Model file for the job. Use its own axes, mm. Give positions to 0.01 mm unless a question says otherwise; leave off trailing zeros. Loops run counter-clockwise (first coordinate to the right, second up) from the corner with the lowest first, then second, coordinate; pieces in that order, holes last. Notation, with made-up numbers: M 65.5,-20.5 L 94.5,-20.5 A23 ccw 94.5,4.5 Z; hole C -27,52 d8. An arc over 180 degrees is marked long. Use CSV: the item, a comma, the result in double quotes. Start each with the question number.
(1) Slice it at A-A on x = 0. List the corners of the cut face in (y, z), and give its area (3 significant figures).
(2) Slice it at B-B on z = -36. List the corners of the cut face in (x, y).
(3) Slice it at C-C on y = 22. List the corners of the cut face in (x, z).
(4) Wall check: line 1 along X through (y, z) = (64.5, 0); line 2 along Z through (x, y) = (54, 66); line 3 along Z through (x, y) = (-15, 9.5). Give the ranges that are in metal, low to high. Write a range as from..to.
(5) Two-plate mould, pull along X, no slides. Class faces 1 (the face through (-1, 99, -456)), 2 (the face through (-51.721, 50.193, -67.453)), 3 (the face through (-100, 49, -355)): pulls with the +X half, pulls with the -X half, needs draft (parallel to the pull), parting line crosses it, or undercut.
```python
from build123d import *

# Parameters (mm, degrees)
BOSS_EXTRUDE1_DEPTH = 99
SKETCH2_R           = 85
CUT_EXTRUDE1_DEPTH  = 99


with BuildPart() as part:
    # Sketch1 → Boss-Extrude1 (new body)
    with BuildSketch(Plane(origin=(0, 0, 0), x_dir=(1, 0, 0), z_dir=(0, 1, 0))):
        with BuildLine():
            ThreePointArc((-100, 0), (0, -100), (100, 0))
            Line((100, 0), (-100, 0))
        make_face()
        with BuildLine():
            Line((-100, 0), (100, 0))
            ThreePointArc((100, 0), (0, 100), (-100, 0))
        make_face()
        with BuildLine():
            ThreePointArc((-100, 0), (0, 100), (100, 0))
            Line((100, 0), (100, 700))
            ThreePointArc((100, 700), (0, 600), (-100, 700))
            Line((-100, 700), (-100, 0))
        make_face()
        with BuildLine():
            ThreePointArc((-100, 700), (0, 600), (100, 700))
            Line((100, 700), (-100, 700))
        make_face()
        with BuildLine():
            Line((-100, 700), (100, 700))
            ThreePointArc((100, 700), (0, 800), (-100, 700))
        make_face()
    extrude(amount=BOSS_EXTRUDE1_DEPTH)

    # Sketch2 → Cut-Extrude1 (cut)
    with BuildSketch(Plane(origin=(0, 99, 0), x_dir=(1, 0, 0), z_dir=(0, 1, 0))):
        with Locations(Location((0, 0, 0), (0, 0, 270))):
            Circle(SKETCH2_R)
    extrude(amount=-CUT_EXTRUDE1_DEPTH, mode=Mode.SUBTRACT)


solid = part.part
```
Reply:
1,outline,"M 0,-800 L 99,-800 L 99,-85 L 0,-85 Z; M 0,85 L 99,85 L 99,100 L 0,100 Z"
1,area,"72,300 mm^2"
2,outline,"M -100,0 L -77,0 L -77,99 L -100,99 Z; M 77,0 L 100,0 L 100,99 L 77,99 Z"
3,outline,"M -100,-700 A100 ccw 100,-700 L 100,0 A100 ccw -100,0 Z; hole C 0,0 d170"
4,line 1,"x = -100..-85, 85..100"
4,line 2,"z = -784.17..-65.64, 65.64..84.17"
4,line 3,"z = -798.87..-83.67, 83.67..98.87"
5,face 1,"needs draft"
5,face 2,"undercut"
5,face 3,"pulls with the -X half"
